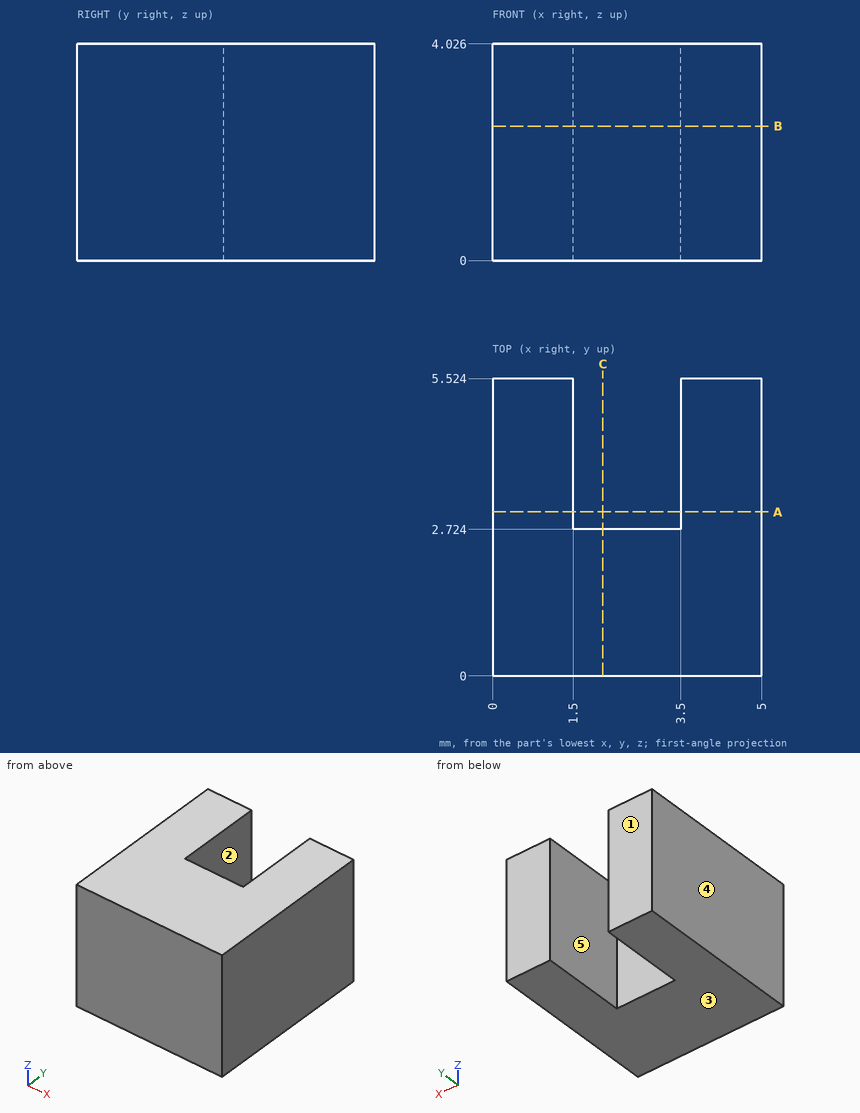
Check sheet for the drawn part. Datum: minimum x, y, z corner. Units: mm. A direction names the side the tool comes from. Round coordinates to 2 decimals unless told otherwise and drop trailing zeros. Order: outer loops, then holes, each group sorted by start corner. A loop starts at its lowest first (then second) coordinate and runs counter-clockwise, first axis right, second up.
1) Go/stop test with a flat-tipped pin: pin 1 Ø1 at (y, z) = (3, 1) entering from -X. Record where the tip stops, or that it passes through.
2) Section check B-B (z = 2.5). Record the boundary of the cut face in (x, y), and give its area (3 significant figures).
3) Section check C-C (x = 2.05). Record the boundary of the cut face in (y, z).
4) Scan lines: line 1 (X direction, y = 4.9, z = 3.4); line 2 (Y direction, x = 1.75, z = 3.6). Record each from-to range of solid material in increasing order.
5) Section check A-A (y = 3.05). Record the boundary of the cut face in (x, z), and give its area (3 significant figures).
6) Mould release check, pull along X, two halves, no side actions. Record for the marked faces 3, 4 and 5: +X half, -X half, draft (parallel to the pull), parting line (faces both ways), or undercut.
7) Tool access check on the marked faces 1 and 2. Record the directions out of +Z, -Z, +X, -X, +Y, -Y that give a thin tool (end or side, any length) a straight path to the whole face; none if there is none.
Result:
1. pin 1: stops at x = 0
2. outline: (0, 0) - (5, 0) - (5, 5.52) - (3.5, 5.52) - (3.5, 2.72) - (1.5, 2.72) - (1.5, 5.52) - (0, 5.52) - close
2. area: 22.0 mm2
3. outline: (0, 0) - (2.72, 0) - (2.72, 4.03) - (0, 4.03) - close
4. line 1: x = 0 to 1.5, 3.5 to 5
4. line 2: y = 0 to 2.72
5. outline: (0, 0) - (1.5, 0) - (1.5, 4.03) - (0, 4.03) - close; (3.5, 0) - (5, 0) - (5, 4.03) - (3.5, 4.03) - close
5. area: 12.1 mm2
6. face 3: draft
6. face 4: -X half
6. face 5: undercut
7. face 1: +Z, -Z, +X, -X, +Y
7. face 2: +Z, -Z, +Y
